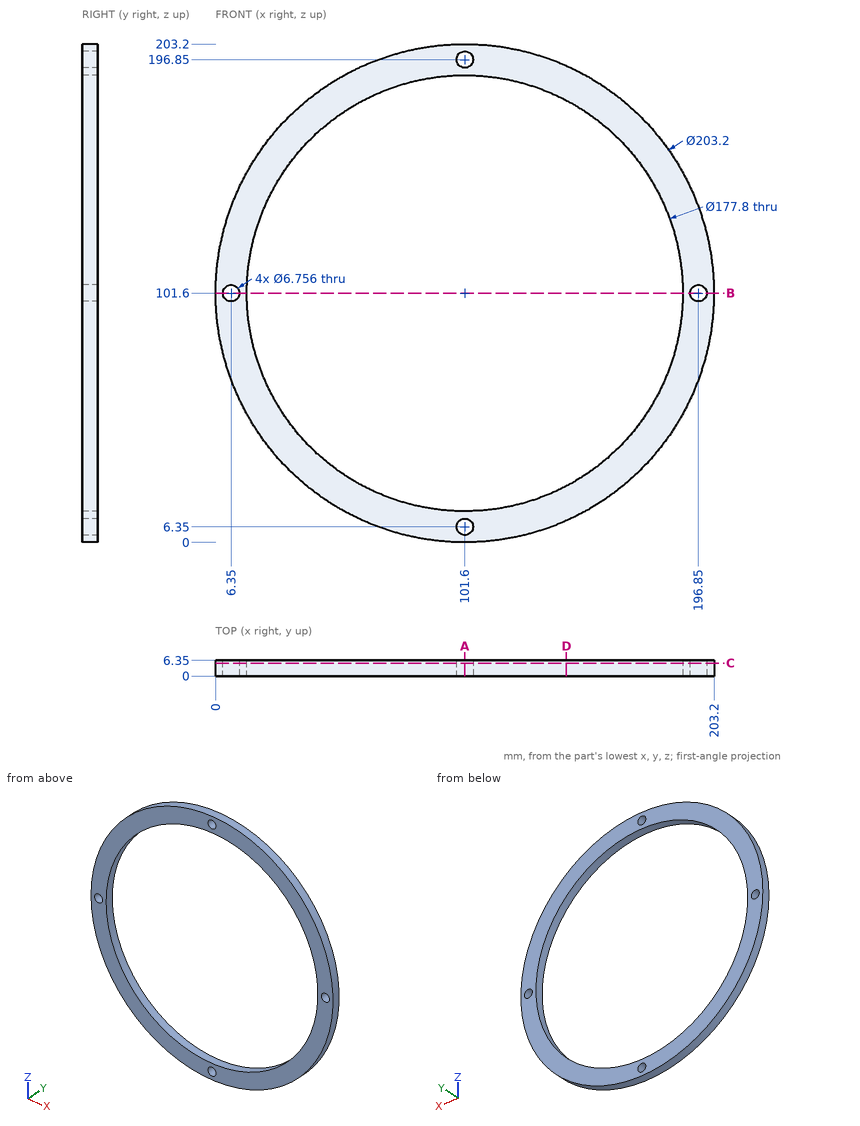
Input: dimensioned drawing with shaded views. Units: mm. Origin: part minimum x, y, z. Give positions to 0.01 mm unless a question says otherwise; leave off trailing zeros. Write each loop counter-clockwise with the first axis right and the second up, starting at its lowest first coordinate (ties: lowest second). Pieces come first, ordered by that corner, then holes. Notation, with made-up numbers: (60, -15.5) -> (97, -15.5) arc R30 ccw to (97, 21.5) -> close; hole circle Ø4 at (62.5, 76). An arc over 180 degrees is marked (long way). Return JSON: item names as keys, results as strings. Group by question number.
1. Section D-D, the plane x = 143. Output: boundary loops of the cut face in (y, z).
2. Pin query (flat end, axial travel): pin 1 Ø2 at (x, y) = (104, 1.5) entering from +Z; pin 2 Ø9 at (x, z) = (196.85, 101.6) entering from -Y; pin 3 Ø1 at (y, z) = (3, 98) entering from +X; pin 4 Ø1 at (x, y) = (163, 1.5) entering from -Z (1 decimal). Return the tip coordinate at first contact, or that it passes through.
3. Section A-A, the plane x = 101.6. Output: boundary loops of the cut face in (y, z).
4. Section B-B, the plane z = 101.6. Output: boundary loops of the cut face in (x, y).
5. Material intervals for line 1 (Z direction, x = 101.6, y = 2); line 2 (Z direction, x = 171, y = 5.5) (1 decimal); line 3 (X direction, y = 3, z = 90) (1 decimal), sorted ascending. Write a range as from..to.
6. Section C-C, the plane y = 5.25. Output: boundary loops of the cut face in (x, z).
Determined:
{
 "1": {"outline": "(0, 8.82) -> (6.35, 8.82) -> (6.35, 22.93) -> (0, 22.93) -> close; (0, 180.27) -> (6.35, 180.27) -> (6.35, 194.38) -> (0, 194.38) -> close"},
 "2": {"pin 1": "stops at z = 203.19", "pin 2": "stops at y = 0", "pin 3": "stops at x = 203.15", "pin 4": "stops at z = 20.3"},
 "3": {"outline": "(0, 0) -> (6.35, 0) -> (6.35, 2.97) -> (0, 2.97) -> close; (0, 9.73) -> (6.35, 9.73) -> (6.35, 12.7) -> (0, 12.7) -> close; (0, 190.5) -> (6.35, 190.5) -> (6.35, 193.47) -> (0, 193.47) -> close; (0, 200.23) -> (6.35, 200.23) -> (6.35, 203.2) -> (0, 203.2) -> close"},
 "4": {"outline": "(0, 0) -> (2.97, 0) -> (2.97, 6.35) -> (0, 6.35) -> close; (9.73, 0) -> (12.7, 0) -> (12.7, 6.35) -> (9.73, 6.35) -> close; (190.5, 0) -> (193.47, 0) -> (193.47, 6.35) -> (190.5, 6.35) -> close; (200.23, 0) -> (203.2, 0) -> (203.2, 6.35) -> (200.23, 6.35) -> close"},
 "5": {"line 1": "z = 0..2.97, 9.73..12.7, 190.5..193.47, 200.23..203.2", "line 2": "z = 27.4..46, 157.2..175.8", "line 3": "x = 0.7..13.5, 189.7..202.5"},
 "6": {"outline": "circle Ø203.2 at (101.6, 101.6); hole circle Ø6.76 at (6.35, 101.6); hole circle Ø177.8 at (101.6, 101.6); hole circle Ø6.76 at (101.6, 6.35); hole circle Ø6.76 at (101.6, 196.85); hole circle Ø6.76 at (196.85, 101.6)"}
}
